from build123d import *

# Parameters (mm, degrees)
BOSS_EXTRUDE1_DEPTH = 28.956
SKETCH2_OUTSIDE_W   = 104.225
SKETCH2_OUTSIDE_H   = 74.976
CUT_EXTRUDE1_DEPTH  = 28.956
CHAMFER1_SIZE       = 17.78
CHAMFER2_SIZE       = 7.62
CHAMFER3_SIZE       = 7.62
SKETCH3_OUTSIDE_W   = 109.871
SKETCH3_OUTSIDE_H   = 49.7
CUT_EXTRUDE2_DEPTH  = 60.198
SKETCH4_OUTSIDE_W   = 48.856
SKETCH4_OUTSIDE_H   = 100.249
CUT_EXTRUDE3_DEPTH  = 65.532


with BuildPart() as part:
    # Sketch1 → Boss-Extrude1 (new body)
    with BuildSketch(Plane.XY):
        with BuildLine():
            add(Edge.make_bspline(
                [(0, 26.329340351), (-15.786544799, 14.596384946), (-36.267616128, 18.74958365)],
                knots=[0, 0, 0, 1, 1, 1], degree=2))
            add(Edge.make_bspline(
                [(-36.267616128, 18.74958365), (-125.980614733, -26.329340351), (0, -26.329340351)],
                knots=[2.349082937, 2.349082937, 2.349082937, 4.702848639, 4.702848639, 4.702848639], degree=2, weights=[1, 0.374957632, 0.976740293]))
            add(Edge.make_bspline(
                [(0, -26.329340351), (0.906326781, -26.329340351), (1.812095783, -26.313136555)],
                knots=[4.702848639, 4.702848639, 4.702848639, 4.747474319, 4.747474319, 4.747474319], degree=2, weights=[0.976740293, 0.988149653, 1]))
            add(Edge.make_bspline(
                [(0, 26.329340351), (15.016751237, 25.038982394), (44.548809621, 18.28020699), (17.807382706, -25.169253325), (1.812095783, -26.313136555)],
                knots=[0, 0, 0, 0, 0.367872962, 0.976947038, 0.976947038, 0.976947038, 0.976947038], degree=3))
        make_face()
    extrude(amount=BOSS_EXTRUDE1_DEPTH)

    # Sketch2 outside → Cut-Extrude1 (cut)
    with BuildSketch(Plane.XY.offset(28.956)):
        with Locations((-10.7055, 0)):
            Rectangle(SKETCH2_OUTSIDE_W, SKETCH2_OUTSIDE_H)
        Polygon((-45.695007292, 8.912831724), (-42.621617043, 12.754569536), (-31.250073118, 12.754569536), (-23.259258469, 12.754569536), (-13.117070645, 16.903646374), (0, 19.055019548), (12.936005686, 21.176695674), (20.690222102, 16.903646374), (23.432684842, 15.392381036), (23.432684842, 8.912831724), (26.072382633, 2.460237124), (22.061453472, -8.912831724), (15.214644669, -17.471342729), (2.473177364, -21.20584876), (-6.558535322, -22.687169165), (-8.760365364, -22.687169165), (-19.88532873, -16.340644797), (-33.401446293, -16.340644797), (-38.472540205, -8.912831724), (-44.158312167, -6.907636041), (-51.519978603, -1.929165251), align=None, mode=Mode.SUBTRACT)
    extrude(amount=-CUT_EXTRUDE1_DEPTH, mode=Mode.SUBTRACT)

    # Chamfer1
    chamfer1_edges = [part.edges().sort_by_distance(p)[0] for p in [
        (-2.042678979, -21.946508963, 28.956),
    ]]
    chamfer(chamfer1_edges, length=CHAMFER1_SIZE)

    # Chamfer2
    chamfer2_edges = [part.edges().sort_by_distance(p)[0] for p in [
        (-18.188164557, 14.829107955, 28.956),
    ]]
    chamfer(chamfer2_edges, length=CHAMFER2_SIZE)

    # Chamfer3
    chamfer3_edges = [part.edges().sort_by_distance(p)[0] for p in [
        (-13.196740008, 12.754569536, 28.956),
    ]]
    chamfer(chamfer3_edges, length=CHAMFER3_SIZE)

    # Sketch3 outside → Cut-Extrude2 (cut)
    with BuildSketch(Plane(origin=(11.964634426, 21.711980874, 0), x_dir=(0.875823084, -0.482632289, 0), z_dir=(0.482632289, 0.875823084, 0))):
        with Locations((-10.7795, -14.478)):
            Rectangle(SKETCH3_OUTSIDE_W, SKETCH3_OUTSIDE_H)
        Polygon((-41.826185128, -14.74462757), (-38.497860604, -21.336), (-35.00576286, -28.251706873), (-26.526762563, -23.970221502), (-15.967663822, -28.251706873), (-9.823064699, -28.251706873), (-3.406709878, -25.011757782), (6.56253296, -26.631732327), (16.221265926, -25.011757782), (21.647404684, -14.478), (23.623550585, -10.068279635), (16.221265926, -2.384533072), (-1.82963065, -2.384533072), (-12.895364261, -7.972193753), (-26.526762563, -5.757129016), (-32.073003248, 0), (-38.436362681, -6.798953713), (-43.484763158, -6.798953713), (-42.326681299, -7.882839769), align=None, mode=Mode.SUBTRACT)
    extrude(amount=-CUT_EXTRUDE2_DEPTH, mode=Mode.SUBTRACT)

    # Sketch4 outside → Cut-Extrude3 (cut)
    with BuildSketch(Plane(origin=(-30.391792793, -20.748992187, 0), x_dir=(0, 0, 1), z_dir=(-0.825881698, -0.563843437, 0))):
        with Locations((14.126, 6.3845)):
            Rectangle(SKETCH4_OUTSIDE_W, SKETCH4_OUTSIDE_H)
        with BuildLine():
            Line((17.379043474, 33.940305121), (20.033797097, 30.011269758))
            Line((20.033797097, 30.011269758), (22.47617043, 30.011269758))
            Line((22.47617043, 30.011269758), (23.108500778, 26.340870516))
            Line((23.108500778, 26.340870516), (27.148536807, 23.108910338))
            Line((27.148536807, 23.108910338), (26.420684971, 19.743661409))
            Line((26.420684971, 19.743661409), (26.420684971, 15.955142831))
            Line((26.420684971, 15.955142831), (26.992031947, 12.638725208))
            Line((26.992031947, 12.638725208), (28.251706873, 7.392768888))
            Line((28.251706873, 7.392768888), (29.39802431, 2.618893435))
            Line((29.39802431, 2.618893435), (28.824865591, -0.031126348))
            Line((28.824865591, -0.031126348), (26.631732327, -2.772601154))
            Line((26.631732327, -2.772601154), (25.821745055, -9.959999212))
            Line((25.821745055, -9.959999212), (23.108500778, -13.351626593))
            Line((23.108500778, -13.351626593), (22.5757173, -18.07926499))
            Line((22.5757173, -18.07926499), (14.257053213, -21.384760387))
            Line((14.257053213, -21.384760387), (11.527022899, -24.797370761))
            Line((11.527022899, -24.797370761), (2.142356235, -22.767611))
            Line((2.142356235, -22.767611), (4.352503323, -18.07926499))
            Line((4.352503323, -18.07926499), (2.384533072, -14.418186985))
            Line((2.384533072, -14.418186985), (2.384533072, -11.501772175))
            Line((2.384533072, -11.501772175), (2.384533072, -1.401863751))
            Line((2.384533072, -1.401863751), (5.601070504, 2.618893435))
            Line((5.601070504, 2.618893435), (5.601070504, 10.015747048))
            Line((5.601070504, 10.015747048), (6.534511478, 14.331544691))
            Line((6.534511478, 14.331544691), (3.992801788, 18.093275032))
            Line((3.992801788, 18.093275032), (1.999794348, 23.108910338))
            Line((1.999794348, 23.108910338), (5.263656633, 27.188824848))
            Line((5.263656633, 27.188824848), (6.798953713, 29.107986959))
            Line((6.798953713, 29.107986959), (8.293414674, 31.975787439))
            Line((8.293414674, 31.975787439), (15.7861913, 31.975787439))
            ThreePointArc((15.7861913, 31.975787439), (16.234438667, 33.24035335), (17.379043474, 33.940305121))
        make_face(mode=Mode.SUBTRACT)
    extrude(amount=-CUT_EXTRUDE3_DEPTH, mode=Mode.SUBTRACT)


solid = part.part
Model file for the job. Use its own axes, mm. A direction names the side the tool comes from. Round coordinates to 2 decimals unless told otherwise and drop trailing zeros. Loops run counter-clockwise (first coordinate to the right, second up) from the corner with the lowest first, then second, coordinate; pieces in that order, holes last. Notation, with made-up numbers: M 70,-37 L 95,-37 A14 ccw 95,-16 Z; hole C 23,22 d8. An arc over 180 degrees is marked long. One line per question, with ' | ' between items.
1) Band-saw the part on C-C (x = -45). Give the cut face in (y, z), then the cut area to 3 significant figures.
Solved:
outline: M -6.34,4.57 L -2.02,6.8 L 4.52,6.8 L 6.53,7.66 L 6.04,7.88 L 5,14.74 L -6.34,25.58 Z | area: 161 mm²
2) Flat gauge pins, fed straight in: pin 1 (12 mm diameter, centred on x = -22, y = 1, fed in from -Z); pin 2 (5.5 mm diameter, centred on x = -39.5, y = -5, fed in from +Z); pin 3 (3 mm diameter, centred on x = -32, z = 8, fed in from -Y). Where does each tip first touch, or does it go through?
Solved:
pin 1: stops at z = 5.88 | pin 2: stops at z = 28.21 | pin 3: stops at y = -16.34
3) Mould opens along X. For faces 5 (the flat face through (4.198, -16.839, 3.382)), 6 (the flat face through (-30, 12.755, 13)), 7 (the flat face through (15.615, -15.934, 13.794)) say: +X half, -X half, draft (parallel to the pull), parting line (faces both ways), or undercut.
Solved:
face 5: undercut | face 6: draft | face 7: +X half
4) Band-saw the part on B-B (z = 17.25). Give the cut face in (x, y).
Solved:
outline: M -48.5,-3.97 L -44.16,-6.91 L -38.47,-8.91 L -33.4,-16.34 L -19.89,-16.34 L -16.65,-18.19 L 16.02,-12.83 L 25.38,4.16 L 23.43,8.91 L 23.43,15.39 L 12.94,21.18 L -13.12,16.9 L -23.26,12.75 L -39.28,12.75 Z
5) Band-saw the part on A-A (x = -28.5). Give the cut face in (y, z).
Solved:
outline: M -16.34,7.29 L -3.5,6.29 L -2.1,6.53 L -1.36,6.12 L 3.24,5.76 L 9.48,2.63 L 12.75,4.8 L 12.75,21.34 L 8.77,25.32 L 3.24,23.97 L -10.58,26.68 L -16.34,20.99 Z
6) Drill centre lines: line 1 along Z through (x, y) = (9, 13); line 2 along Z through (x, y) = (-20, -12); line 3 along Y through (x, z) = (2, 11.25). Where is each one in solid material? Low to high.
Solved:
line 1: z = 5.6 to 25.83 | line 2: z = 7.38 to 23.9 | line 3: y = -21.21 to 19.38
7) 3-axis set-ups, long thin cutter, end or side, ignore diameter. For faces 1 (the flat face through (-28.78, 5.61, 4.32)), 2 (the flat face through (-10.917, 9.44, 26.766)), 3 (the flat face through (-39, -4, 26.421)), 4 (the flat face through (-34.128, -7.133, 6.323)): which of +Z, -Z, +X, -X, +Y, -Y reach the whole face in a straight line?
Solved:
face 1: -Z, -Y | face 2: +Z, +Y | face 3: +Z | face 4: -Z
